Check sheet for the modelled part. Datum: model origin and axes. Units: mm. Face numbers are marked on the shaded views. A direction names the side the tool comes from. Give positions to 0.01 mm unless a question says otherwise; leave off trailing zeros. Write each loop counter-clockwise with the first axis right and the second up, starting at its lowest first coordinate (ties: lowest second). Pieces come first, ordered by that corner, then holes. Notation, with made-up numbers: (31.25, 35) - (52.25, 35) arc R15 cw to (52.25, 52) - close; hole circle Ø8 at (4, 36). An arc over 180 degrees is marked (long way). Return JSON: item names as keys, results as strings. Group by question number.
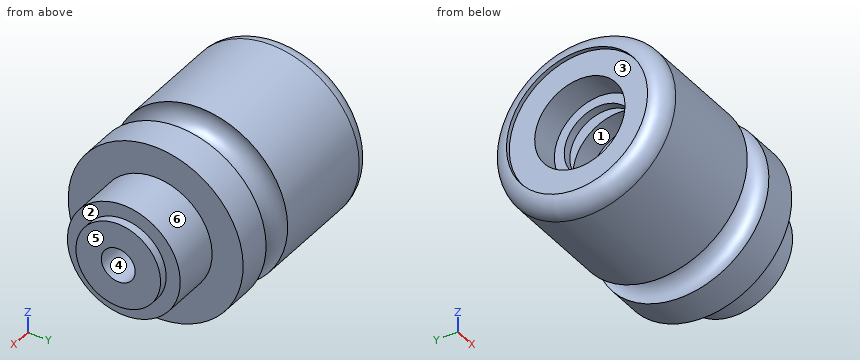
```python
from build123d import *

# Parameters (mm, degrees)
F4_R = 5.99999


# Not quite as in the source:
# - a fillet or chamfer is up to 0.001 mm smaller than in the source, because OpenCascade refuses the exact size


with BuildPart() as f1:
    # F0 (on Front) → F1 (revolve)
    with BuildSketch(Plane.XZ):
        with BuildLine():
            Line((0, 31), (0, 0))
            Line((0, 0), (88, 0))
            Line((88, 0), (88, 15))
            Line((88, 15), (85, 15))
            Line((85, 15), (85, 20))
            Line((85, 20), (68, 20))
            Line((68, 20), (68, 31))
            Line((68, 31), (55.7656139637, 31))
            ThreePointArc((55.7656139637, 31), (50, 23.3393689087), (44.2343860363, 31))
            Line((44.2343860363, 31), (0, 31))
        make_face()
    revolve(axis=Axis((85.9634177689, 0, 0), (1, 0, 0)))

    # F2 (on Front) → F3 (revolve, cut)
    with BuildSketch(Plane.XZ):
        Polygon((0, 25), (0, 0), (88, 0), (88, 6), (30, 6), (30, 12.5), (30, 16), (22, 16), (22, 20.5), (15, 20.5), (15, 12.5), (12, 12.5), (12, 16), (1.5, 16), (1.5, 25), align=None)
    revolve(axis=Axis((-10.4486994627, 0, 0), (-1, 0, 0)), mode=Mode.SUBTRACT)

    # F4 (radius 6 in the source; OpenCascade refuses exactly that, so slightly less here)
    f4_edges = [f1.edges().sort_by_distance(p)[0] for p in [
        (0, 0, -31),
    ]]
    fillet(f4_edges, radius=F4_R)


solid = f1.part
```
Item 1: Section check A-A on x = 18.5. Record the cut outline in (y, z), plus the area to 3 significant figures.
Item 2: Depth check by flat-ended pin: pin 1 (3 mm diameter, centred on x = 47, z = -7, fed in from -Y); pin 2 (12.5 mm diameter, centred on y = 1.5, z = -2.5, fed in from -X); pin 3 (2 mm diameter, centred on y = -1.5, z = 19.5, fed in from +X). Enter the tip coordinate at first touch or a pass-through.
Item 3: Material ranges on line 1 along X through (y, z) = (-12.5, -15); line 2 along Y through (x, z) = (72, 2.5); line 3 along X through (y, z) = (-19, 13.5), recorded low to high. Write a range as from..to.
Item 4: Access from +Z, -Z, +X, -X, +Y, -Y to the whole of each face (thin tool, end or side, straight path). Record for the marked faces 1, 2 and 3.
Item 5: Mould release check, pull along Y, two halves, no side actions. Record for the marked faces 4, 5 and 6: +Y half, -Y half, draft (parallel to the pull), parting line (faces both ways), or undercut.
Item 6: Section check B-B on x = 77.5. Record the cut outline in (y, z).
Reply:
{
 "1": {"outline": "circle Ø62 at (0, 0); hole circle Ø41 at (0, 0)", "area": "1,700 mm²"},
 "2": {"pin 1": "y = -24.44", "pin 2": "x = 30", "pin 3": "x = 85"},
 "3": {"line 1": "1.5..15, 22..85", "line 2": "-19.84..-5.45, 5.45..19.84", "line 3": "1.5..68"},
 "4": {"face 1": "none", "face 2": "+X", "face 3": "-X"},
 "5": {"face 4": "undercut", "face 5": "draft", "face 6": "parting line"},
 "6": {"outline": "circle Ø40 at (0, 0); hole circle Ø12 at (0, 0)"}
}
